Source: CAD feature listing. Evaluate the final solid. Frame: model axes, mm. Face numbers are marked on the shaded views. Give positions to 0.01 mm unless a question says otherwise; leave off trailing zeros. Loops run counter-clockwise (first coordinate to the right, second up) from the corner with the lowest first, then second, coordinate; pieces in that order, holes last. Notation, with made-up numbers: M -36,-29 L -32,-29 A27 ccw -32,0 Z; hole C 51.25,16 d10. An arc over 180 degrees is marked long. Put each result on its own line as item: value. Start each with the question number.
Autodesk Inventor part; units mm, degrees
ref_plane "YZ Plane" through (0, 0, 0) normal (1, 0, 0) x (0, 1, 0)
ref_plane "XZ Plane" through (0, 0, 0) normal (0, 1, 0) x (-1, 0, 0)
ref_plane "XY Plane" through (0, 0, 0) normal (0, 0, 1) x (1, 0, 0)
sketch "washer_sketch" plane through (0, 0, 0) normal (0, 0, 1) x (1, 0, 0)
  arc A0 (0.0668, 4.8898) -> (-1.1152, 4.3995) centre (0.2018, 2.8944) ccw construction
  line L0 (-7.8667, -1.508) -> (-1.1152, 4.3995) construction
  arc A1 (-7.8667, -1.508) -> (-8.5497, -3.0131) centre (-6.5497, -3.0131) ccw construction
  line L1 (-8.5497, -4.8898) -> (-8.5497, -3.0131) construction
  line L2 (8.5497, -4.8898) -> (-8.5497, -4.8898) construction
  line L3 (1.5081, 4.1255) -> (8.5497, -4.8898) construction
  arc A2 (1.5081, 4.1255) -> (0.0668, 4.8898) centre (-0.0681, 2.8944) ccw construction
  circle A3 centre (-0.4046, -0.6987) radius 3.55 construction
  circle A4 centre (-0.4046, -0.6987) radius 3.55 construction
  circle A5 centre (-0.4046, -0.6987) radius 1.4
  line L4 (-6.4046, -4.8898) -> (5.5954, -4.8898)
  line L5 (7.5954, -2.8898) -> (7.5954, 1.4924)
  line L6 (5.5954, 3.4924) -> (-6.4046, 3.4924)
  line L7 (-8.4046, 1.4924) -> (-8.4046, -2.8898)
  arc A6 (-8.4046, -2.8898) -> (-6.4046, -4.8898) centre (-6.4046, -2.8898) ccw
  arc A7 (-6.4046, 3.4924) -> (-8.4046, 1.4924) centre (-6.4046, 1.4924) ccw
  arc A8 (7.5954, 1.4924) -> (5.5954, 3.4924) centre (5.5954, 1.4924) ccw
  arc A9 (5.5954, -4.8898) -> (7.5954, -2.8898) centre (5.5954, -2.8898) ccw
  point P0 (0, 0)
  point P1 (-8.4046, -4.8898)
  point P2 (7.5954, 3.4924)
  point P3 (-8.4046, 3.4924)
  dimension "d0" = 16
  dimension "d1" = 8
  dimension "d2" = 4.1911
  dimension "d3" = 4.1911
  dimension "d4" = 2
extrude "washer" add sketch "washer_sketch" along normal blind 2
equation "\"d1\" = 0.5 * d0"
equation "\"d3\" = d2"
properties part number "mount_linear_stepper_washer"
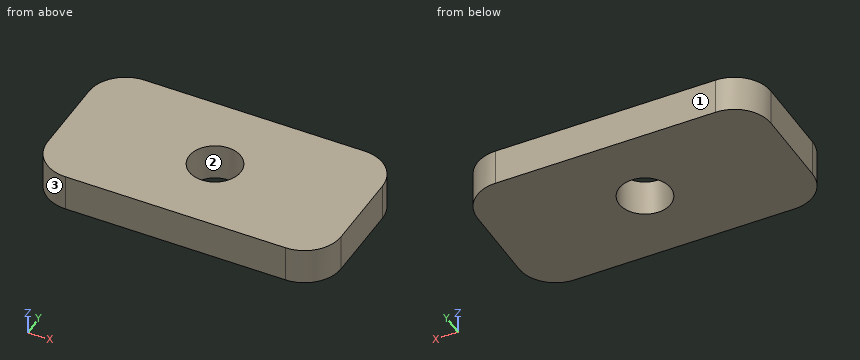
1. Section B-B, the plane z = 0.5. Output: boundary loops of the cut face in (x, y).
2. Section D-D, the plane y = -4. Output: boundary loops of the cut face in (x, z), plus the area to 3 significant figures.
3. Contact query for a flat-ended pin moving along its axis: pin 1 (3 mm diameter, centred on x = -3.5, y = -1.5, fed in from -Z). Output: stop coordinate, or through.
4. Ray query, line 1 (X direction, y = -0.5, z = 0.35); line 2 (Y direction, x = -0.75, z = 1.05); line 3 (X direction, y = -3, z = 1.8). Return the intervals inside material, ascending.
5. Pull-direction query (X, two-part tool) for the marked faces 1, 2 and 3; classes: released by +X, released by -X, zero draft, split by the parting line, or undercut.
6. Section A-A, the plane y = 0.5. Output: boundary loops of the cut face in (x, z), plus the area to 3 significant figures.
7. Section C-C, the plane x = -0.25. Output: boundary loops of the cut face in (y, z), plus the area to 3 significant figures.
Results found:
1. outline: M -8.4,-2.89 A2 ccw -6.4,-4.89 L 5.6,-4.89 A2 ccw 7.6,-2.89 L 7.6,1.49 A2 ccw 5.6,3.49 L -6.4,3.49 A2 ccw -8.4,1.49 Z; hole C -0.4,-0.7 d2.8
2. outline: M -8.07,0 L 7.26,0 L 7.26,2 L -8.07,2 Z
2. area: 30.7 mm²
3. pin 1: z = 0
4. line 1: -8.4 to -1.79, 0.98 to 7.6
4. line 2: -4.89 to -2.06, 0.66 to 3.49
4. line 3: -8.4 to 7.59
5. face 1: zero draft
5. face 2: undercut
5. face 3: released by -X
6. outline: M -8.4,0 L -1.13,0 L -1.13,2 L -8.4,2 Z; M 0.32,0 L 7.6,0 L 7.6,2 L 0.32,2 Z
6. area: 29.1 mm²
7. outline: M -4.89,0 L -2.09,0 L -2.09,2 L -4.89,2 Z; M 0.69,0 L 3.49,0 L 3.49,2 L 0.69,2 Z
7. area: 11.2 mm²
